Read the model definition and answer for the solid it produces. Units are mm, in the model's axes. A direction names the side the tool comes from. Round coordinates to 2 decimals unless told otherwise and drop trailing zeros. Order: outer loops, then holes, each group sorted by start corner. A loop starts at its lowest first (then second) coordinate and runs counter-clockwise, first axis right, second up. Notation, with made-up numbers: (31, -1.5) -> (85, -1.5) arc R24 cw to (85, 24.5) -> close; hole circle Ø9 at (-17, 36.25). An arc over 180 degrees is marked (long way). Use a Markdown table: item, result. Add a question column.
1. Consider L1, parallel to X at y = -56.75, z = 91.5; L2, parallel to Z at x = 8.5, y = -58 (3 decimals); L3, parallel to Y at x = 3, z = 127. Determine where each line is inside the solid, lowest interval first. Write a range as [from, to].
2. Section C-C, the plane x = 2.5 is taken. Give the vertices of the cut face in (y, z) (3 decimals).
3. Given pin 1 (1 mm diameter, centred on x = -29.5, y = -57, fed in from +Z) (3 decimals); pin 2 (1 mm diameter, centred on x = -15, z = 138.5, fed in from +Y), each flat-ended and moving along its own axis, determine where each tip first touches the part or whether it passes through.
4. Section B-B, the plane z = 120 is taken. Give the vertices of the cut face in (x, y), then the cut area to 3 significant figures.
5. For faces 4 (the face through (-25, -58, 3.175)), 5 (the face through (-24, -63, 222.25)), determine the directions among +Z, -Z, +X, -X, +Y, -Y from which every point of the face is accessible in a straight line to the end or side of a thin tool.
6. The mould has two halves that part along X. Classify faces 1 (the face through (-85.248, -60, 110)), 2 (the face through (-25, -62.739, 111)), 3 (the face through (-25, -65.914, 110)): +X half, -X half, draft (parallel to the pull), parting line (faces both ways), or undercut.
```python
from build123d import *

# Parameters (mm, degrees)
SKETCH2_W           = 122.201758268
SKETCH2_H           = 12.52058784
BOSS_EXTRUDE1_DEPTH = 222.25
SHELL1_T            = -3.175


with BuildPart() as part:
    # Sketch2 → Boss-Extrude1 (new body)
    with BuildSketch(Plane.XY):
        with Locations((-24.147384347, -59.653504879)):
            Rectangle(SKETCH2_W, SKETCH2_H)
    extrude(amount=BOSS_EXTRUDE1_DEPTH)

    # Shell1
    shell1_openings = [part.faces().sort_by_distance(p)[0] for p in [
        (-24.147384347, -59.653504879, 222.25),
        (-24.147384347, -53.393210959, 111.125),
    ]]
    offset(amount=SHELL1_T, openings=shell1_openings, kind=Kind.INTERSECTION)


solid = part.part
```
Verdict:
| question | item | result |
|---|---|---|
| 1 | L1 | x = [-85.25, -82.07], [33.78, 36.95] |
| 1 | L2 | z = [0, 3.175] |
| 1 | L3 | y = [-65.91, -62.74] |
| 2 | outline | (-65.914, 0) -> (-53.393, 0) -> (-53.393, 3.175) -> (-62.739, 3.175) -> (-62.739, 222.25) -> (-65.914, 222.25) -> close |
| 3 | pin 1 | stops at z = 3.175 |
| 3 | pin 2 | stops at y = -62.74 |
| 4 | outline | (-85.25, -65.91) -> (36.95, -65.91) -> (36.95, -53.39) -> (33.78, -53.39) -> (33.78, -62.74) -> (-82.07, -62.74) -> (-82.07, -53.39) -> (-85.25, -53.39) -> close |
| 4 | area | 447 mm2 |
| 5 | face 4 | +Z, +Y |
| 5 | face 5 | +Z, +X, -X, +Y, -Y |
| 6 | face 1 | -X half |
| 6 | face 2 | undercut |
| 6 | face 3 | draft |
